```python
from build123d import *

# Parameters (mm, degrees)
F1_DEPTH = 25.4


with BuildPart() as f1:
    # F0 (on Front) → F1 (new body)
    with BuildSketch(Plane.XZ):
        with BuildLine():
            ThreePointArc((-37.2795093382, 40.0635529992), (-37.0944265378, 41.8428324334), (-37.0326339638, 43.6306446791))
            ThreePointArc((-37.0326339638, 43.6306446791), (-37.0352597257, 43.9993926792), (-37.0431364787, 44.3680658937))
            Line((-37.0431364787, 44.3680658937), (-59.2393539846, 44.3680658937))
            Line((-59.2393539846, 44.3680658937), (-59.2393539846, 34.8789981649))
            ThreePointArc((-59.2393539846, 34.8789981649), (-48.6715325086, 39.2167813917), (-37.2795093382, 40.0635529992))
        make_face()
        with BuildLine():
            ThreePointArc((-37.0431364787, 44.3680658937), (-37.0352597257, 43.9993926792), (-37.0326339638, 43.6306446791))
            ThreePointArc((-37.0326339638, 43.6306446791), (-37.0944265378, 41.8428324334), (-37.2795093382, 40.0635529992))
            ThreePointArc((-37.2795093382, 40.0635529992), (-36.8032339812, 40.0205567646), (-36.3275649384, 39.9713038099))
            ThreePointArc((-36.3275649384, 39.9713038099), (-36.5428213794, 42.1645221032), (-36.573424985, 44.3680658936))
            Line((-36.573424985, 44.3680658937), (-37.0431364787, 44.3680658937))
        make_face()
        with BuildLine():
            Line((-59.2393539846, 44.3680658937), (-37.0431364787, 44.3680658937))
            ThreePointArc((-37.0431364787, 44.3680658937), (-77.5434180545, 65.0043168763), (-73.0012082171, 19.7771569817))
            ThreePointArc((-73.0012082171, 19.7771569817), (-67.2022274173, 28.3140227514), (-59.2393539846, 34.8789981649))
            Line((-59.2393539846, 34.8789981649), (-59.2393539846, 44.3680658937))
        make_face()
        with BuildLine():
            ThreePointArc((-36.3275649384, 39.9713038099), (-36.8032339812, 40.0205567646), (-37.2795093382, 40.0635529992))
            ThreePointArc((-37.2795093382, 40.0635529992), (-44.4588292576, 25.4802541483), (-58.915556877, 18.0493547131))
            Line((-58.915556877, 18.0493547131), (-16.2551814161, 18.0493547131))
            ThreePointArc((-16.2551814161, 18.0493547131), (-29.6914752573, 25.897095458), (-36.3275649384, 39.9713038099))
        make_face()
        with BuildLine():
            ThreePointArc((-58.915556877, 18.0493547131), (-44.4588292576, 25.4802541483), (-37.2795093382, 40.0635529992))
            ThreePointArc((-37.2795093382, 40.0635529992), (-48.6715325086, 39.2167813917), (-59.2393539846, 34.8789981649))
            Line((-59.2393539846, 34.8789981649), (-59.2393539846, 18.0493547131))
            Line((-59.2393539846, 18.0493547131), (-58.915556877, 18.0493547131))
        make_face()
        with BuildLine():
            ThreePointArc((-59.2393539846, 34.8789981649), (-67.2022274173, 28.3140227514), (-73.0012082171, 19.7771569817))
            ThreePointArc((-73.0012082171, 19.7771569817), (-66.0790584232, 17.9294636931), (-58.915556877, 18.0493547131))
            Line((-58.915556877, 18.0493547131), (-59.2393539846, 18.0493547131))
            Line((-59.2393539846, 18.0493547131), (-59.2393539846, 34.8789981649))
        make_face()
        with BuildLine():
            ThreePointArc((-58.915556877, 18.0493547131), (-66.0790584232, 17.9294636931), (-73.0012082171, 19.7771569817))
            ThreePointArc((-73.0012082171, 19.7771569817), (-48.5063899421, -31.6353638875), (-3.9320745419, 3.8100001402))
            ThreePointArc((-3.9320745419, 3.8100001402), (-4.620150317, 10.8521017976), (-6.6583498303, 17.6278221851))
            ThreePointArc((-6.6583498303, 17.6278221851), (-11.4762045796, 17.3960309275), (-16.2551814161, 18.0493547131))
            Line((-16.2551814161, 18.0493547131), (-58.915556877, 18.0493547131))
        make_face()
        with BuildLine():
            Line((-16.2551814161, 44.3680658937), (-36.573424985, 44.3680658937))
            ThreePointArc((-36.573424985, 44.3680658936), (-36.5428213794, 42.1645221032), (-36.3275649384, 39.9713038099))
            ThreePointArc((-36.3275649384, 39.9713038099), (-25.6065541108, 37.085516119), (-16.2551814161, 31.1005622773))
            Line((-16.2551814161, 31.1005622773), (-16.2551814161, 44.3680658937))
        make_face()
        with BuildLine():
            ThreePointArc((15.9360373073, 43.6306446791), (-9.9551248939, 69.8879647074), (-36.573424985, 44.3680658936))
            Line((-36.573424985, 44.3680658937), (-16.2551814161, 44.3680658937))
            Line((-16.2551814161, 44.3680658937), (-16.2551814161, 31.1005622773))
            ThreePointArc((-16.2551814161, 31.1005622773), (-10.6808873976, 24.916861741), (-6.6583498303, 17.6278221851))
            ThreePointArc((-6.6583498303, 17.6278221851), (9.4983266183, 26.4067288367), (15.9360373073, 43.6306446791))
        make_face()
        with BuildLine():
            ThreePointArc((-16.2551814161, 31.1005622773), (-25.6065541108, 37.085516119), (-36.3275649384, 39.9713038099))
            ThreePointArc((-36.3275649384, 39.9713038099), (-29.6914752573, 25.897095458), (-16.2551814161, 18.0493547131))
            Line((-16.2551814161, 18.0493547131), (-16.2551814161, 31.1005622773))
        make_face()
        with BuildLine():
            Line((-16.2551814161, 31.1005622773), (-16.2551814161, 18.0493547131))
            ThreePointArc((-16.2551814161, 18.0493547131), (-11.4762045796, 17.3960309275), (-6.6583498303, 17.6278221851))
            ThreePointArc((-6.6583498303, 17.6278221851), (-10.6808873976, 24.916861741), (-16.2551814161, 31.1005622773))
        make_face()
    extrude(amount=F1_DEPTH)


solid = f1.part
```
Geometry: final body of the model. Coordinates: model frame, mm. Round coordinates to 2 decimals unless told otherwise and drop trailing zeros. Write each loop counter-clockwise with the first axis right and the second up, starting at its lowest first coordinate (ties: lowest second). Pieces come first, ordered by that corner, then holes. Notation, with made-up numbers: M 86,-34 L 111,-34 A20 ccw 111,-6 Z; hole C 14,-28.5 d3. An arc over 180 degrees is marked long. Answer in a Markdown table with one row per item. Add a question column.
(1) Ray query, L1, parallel to X at y = -14.25, z = 63.5; L2, parallel to Z at x = -10.5, y = -18.5; L3, parallel to X at y = -17.25, z = 51. Return the intervals inside material, ascending.
(2) Draft query along X for faces 1 (the face through (-37, 0, 19)), 2 (the face through (-76.9, -12.52, 65.43)). Return one class per face: pulls with the +X half, pulls with the -X half, needs draft (parallel to the pull), parting line crosses it, or undercut.
(3) Cut plane C-C, the plane x = -33. Return the cut outline in (y, z), then the cut area to 3 significant figures.
(4) Cut plane B-B, the plane y = -11.25. Return the cut outline in (x, z).
(5) Contact query for flat-ended pins moving along their axis: pin 1 (10 mm diameter, centred on x = -53.5, y = -5, fed in from +Z); pin 2 (1 mm diameter, centred on x = -26.5, z = 22, fed in from +Y); pin 3 (10 mm diameter, centred on y = -17, z = 49, fed in from -X); pin 4 (1 mm diameter, centred on x = -75, y = -21.5, fed in from +Z). Output: stop coordinate, or through.
(6) Cut plane A-A, the plane z = 47.5. Return the cut outline in (x, y), then the cut area to 3 significant figures.
(7) Cut plane D-D, the plane z = 9. Return the cut outline in (x, y).
Established:
| question | item | result |
|---|---|---|
| 1 | L1 | -79.53 to -46.32, -27.49 to 6.85 |
| 1 | L2 | -17.04 to 69.89 |
| 1 | L3 | -87.75 to -38.1, -35.53 to 14.88 |
| 2 | face 1 | needs draft |
| 2 | face 2 | undercut |
| 3 | outline | M -25.4,-31.83 L 0,-31.83 L 0,56.87 L -25.4,56.87 Z |
| 3 | area | 2,250 mm² |
| 4 | outline | M -73,19.78 A36.38 ccw long -6.66,17.63 A26.26 ccw long -36.57,44.37 L -37.04,44.37 A25.89 ccw long Z |
| 5 | pin 1 | z = 69.14 |
| 5 | pin 2 | y = 0 |
| 5 | pin 3 | x = -88.82 |
| 5 | pin 4 | z = 66.79 |
| 6 | outline | M -88.53,-25.4 L -37.32,-25.4 L -37.32,0 L -88.53,0 Z; M -36.3,-25.4 L 15.65,-25.4 L 15.65,0 L -36.3,0 Z |
| 6 | area | 2,620 mm² |
| 7 | outline | M -76.32,-25.4 L -4.3,-25.4 L -4.3,0 L -76.32,0 Z |
